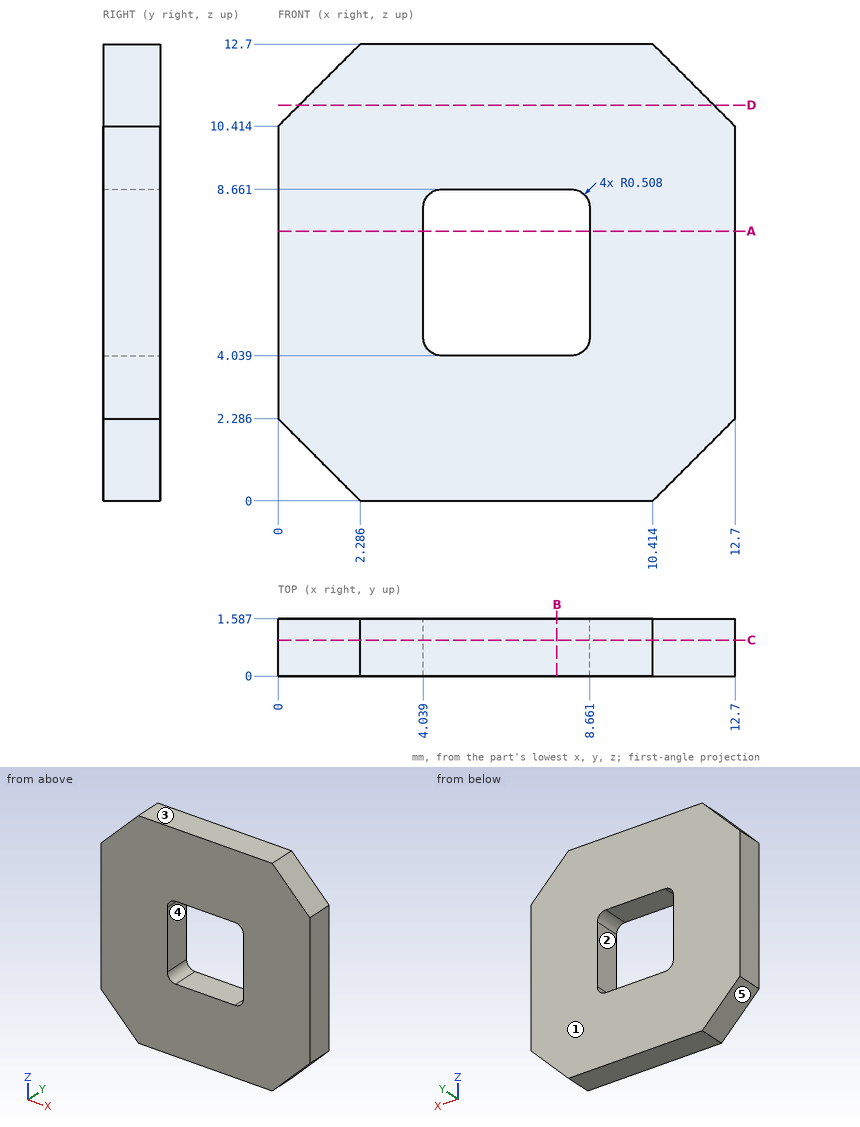
Check sheet for the drawn part. Datum: minimum x, y, z corner. Units: mm. A direction names the side the tool comes from. Round coordinates to 2 decimals unless told otherwise and drop trailing zeros. Write each loop counter-clockwise with the first axis right and the second up, starting at its lowest first coordinate (ties: lowest second). Pieces come first, ordered by that corner, then holes. Notation, with made-up numbers: (-13.75, 32) - (29.25, 32) arc R23 ccw to (29.25, 64) - close; hole circle Ø7 at (-3, 31). An arc over 180 degrees is marked (long way). Write each question's results on one line, items separated by ' | '.
(1) Sectioned sample at D-D, the plane z = 11. Enter the section's corners in (x, y) (1 decimal).
Computed:
outline: (0.6, 0) - (12.1, 0) - (12.1, 1.6) - (0.6, 1.6) - close
(2) Set-up check for the marked faces 1 and 2: record each of +Z, -Z, +X, -X, +Y, -Y from which the full face is reachable in a straight line by a thin tool's end or side.
Computed:
face 1: +Z, -Z, +X, -X, +Y | face 2: +Y, -Y
(3) Sectioned sample at B-B, the plane x = 7.75. Enter the section's corners in (y, z), plus the area to 3 significant figures.
Computed:
outline: (0, 0) - (1.59, 0) - (1.59, 4.04) - (0, 4.04) - close; (0, 8.66) - (1.59, 8.66) - (1.59, 12.7) - (0, 12.7) - close | area: 12.8 mm^2
(4) Sectioned sample at A-A, the plane z = 7.5. Enter the section's corners in (x, y), plus the area to 3 significant figures.
Computed:
outline: (0, 0) - (4.04, 0) - (4.04, 1.59) - (0, 1.59) - close; (8.66, 0) - (12.7, 0) - (12.7, 1.59) - (8.66, 1.59) - close | area: 12.8 mm^2
(5) Sectioned sample at C-C, the plane y = 1. Enter the section's corners in (x, z) (1 decimal), plus the area to 3 significant figures.
Computed:
outline: (0, 2.3) - (2.3, 0) - (10.4, 0) - (12.7, 2.3) - (12.7, 10.4) - (10.4, 12.7) - (2.3, 12.7) - (0, 10.4) - close; hole (4, 4.5) arc R0.5 ccw to (4.5, 4) - (8.2, 4) arc R0.5 ccw to (8.7, 4.5) - (8.7, 8.2) arc R0.5 ccw to (8.2, 8.7) - (4.5, 8.7) arc R0.5 ccw to (4, 8.2) - close | area: 130 mm^2
(6) Draft check along X on the marked faces 3, 4 and 5. Enter one of: pulls with the +X half, pulls with the -X half, needs draft (parallel to the pull), parting line crosses it, or undercut.
Computed:
face 3: needs draft | face 4: undercut | face 5: pulls with the -X half
(7) Thickness scan on probe 1 along Z at (x, y) = (8, 1.5); probe 2 along X at (y, z) = (1.45, 11.5) (1 decimal). Record the ranges inside material, lowest first. Write a range as from..to.
Computed:
probe 1: z = 0..4.04, 8.66..12.7 | probe 2: x = 1.1..11.6
